Input: part model. Units: mm. Frame: model coordinates. Face numbers are marked on the shaded views. A direction names the side the tool comes from. Coordinates: 2 decimals unless noted, no trailing zeros. Order: outer loops, then holes, each group sorted by start corner. A loop starts at its lowest first (then second) coordinate and runs counter-clockwise, first axis right, second up. Notation, with made-up numbers: (3.5, -28.75) -> (30.5, -28.75) arc R18 ccw to (30.5, -16.75) -> close; hole circle Ø7 at (20.5, 5). An arc over 180 degrees is marked (long way). One line per item, written item: value. Start each with the question number.
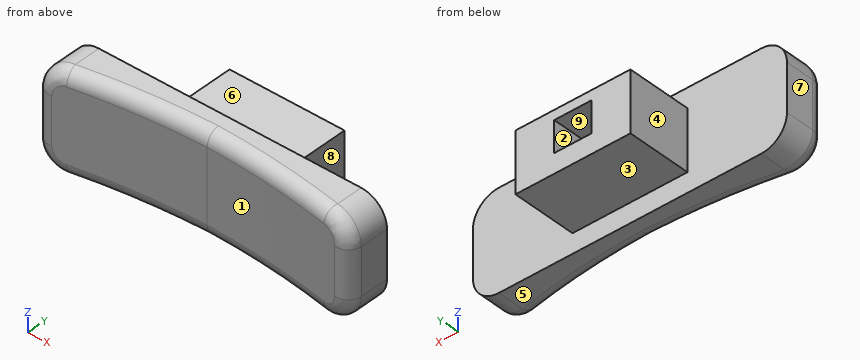
Autodesk Inventor part; units mm, degrees
ref_plane "Work Plane1" through (65.3719, 0, -59.3656) normal (0, 0, -1) x (-1, 0, 0)
ref_plane "Work Plane2" through (64.6469, 0, -58.7656) normal (1, 0, 0) x (0, 0, -1)
ref_plane "YZ Plane" through (0, 0, 0) normal (1, 0, 0) x (0, 1, 0)
sketch "Sketch3" plane through (0, 0, 0) normal (0, 1, 0) x (-1, 0, 0)
  line L0 (-64.0219, -58.8656) -> (-65.2719, -58.8656)
  line L1 (-65.2719, -58.8656) -> (-65.2719, -59.8656)
  line L2 (-65.2719, -59.8656) -> (-64.0219, -59.8656)
  line L3 (-64.0219, -59.8656) -> (-64.0219, -58.8656)
  line L4 (-63.9219, -59.9656) -> (-65.3719, -59.9656)
  line L5 (-65.3719, -59.9656) -> (-65.3719, -58.7656)
  line L6 (-65.3719, -58.7656) -> (-63.9219, -58.7656)
  line L7 (-63.9219, -58.7656) -> (-63.9219, -59.9656)
  line L8 (-66.8719, -60.7156) -> (-62.4219, -60.7156)
  line L9 (-62.4219, -60.7156) -> (-62.4219, -58.3956)
  line L10 (-62.4219, -58.3956) -> (-66.8719, -58.3956)
  line L11 (-66.8719, -58.3956) -> (-66.8719, -60.7156)
  line L12 (-70.1719, -61.0956) -> (-70.1719, -58.0956)
  line L13 (-70.1719, -58.0956) -> (-60.6119, -58.0956)
  line L14 (-60.6119, -61.0956) -> (-60.6119, -58.0956)
  dimension "d4" = 0.1
  dimension "d8" = 1.5
  dimension "d9" = 1.5
  dimension "d10" = 0.3
  dimension "d11" = 0.75
extrude "Extrusion3" add sketch "Sketch3" along normal blind 2.5 contours L11 L10 L9 L8
ref_plane "Work Plane1" through (65.3719, 0, -59.3656) normal (0, 0, -1) x (-1, 0, 0)
ref_plane "Work Plane2" through (64.6469, 0, -58.7656) normal (1, 0, 0) x (0, 0, -1)
sketch "Sketch4" plane through (0, 0, 0) normal (0, -1, 0) x (1, 0, 0)
  line L0 (60.1219, -61.0956) -> (60.1219, -58.0956)
  line L1 (67.6819, -58.0956) -> (67.6819, -61.0956)
  line L2 (60.1219, -58.0956) -> (67.6819, -58.0956)
  line L3 (62.4219, -58.3956) -> (66.8719, -58.3956)
  line L4 (66.8719, -58.3956) -> (66.8719, -60.7156)
  line L5 (66.8719, -60.7156) -> (62.4219, -60.7156)
  line L6 (62.4219, -60.7156) -> (62.4219, -58.3956)
  line L7 (70.7219, -57.6456) -> (58.5719, -57.6456)
  line L8 (58.5719, -57.6456) -> (58.5719, -61.4656)
  line L9 (58.5719, -61.4656) -> (70.7219, -61.4656)
  line L10 (70.7219, -61.4656) -> (70.7219, -57.6456)
  dimension "d13" = 3.85
  dimension "d14" = 3.85
extrude "Extrusion4" add sketch "Sketch4" along normal blind 1 contours L3 L4 L5 L6 | L10 L9 L8 L7
fillet "Fillet1" radius 1 4 edges at (70.7219, -0.5, -61.4656) (58.5719, -0.5, -61.4656) (58.5719, -0.5, -57.6456) (70.7219, -0.5, -57.6456)
sketch "Sketch6" plane through (69.7219, 0, -61.4656) normal (0, 0, -1) x (-1, 0, 0)
  line L0 (10.15, -1) -> (0, -1)
  line L1 (11.15, -1) -> (10.15, -1)
  line L2 (0, -1) -> (-1, -1)
  line L3 (11.15, -1) -> (11.15, -1.75)
  line L4 (0, -1) -> (10.15, -1)
  line L5 (5.075, -1) -> (5.075, -2.2009)
  arc A0 (11.15, -1.75) -> (5.075, -1) centre (4.574, -30.0368) ccw
  line L6 (-1, -1) -> (-1, -1.75)
  arc A1 (5.075, -1) -> (-1, -1.75) centre (5.576, -30.0368) ccw
  dimension "d18" = 0.75
extrude "Extrusion5" add sketch "Sketch6" against normal up to surface (3.82 mm away)
sketch "Sketch7" plane through (69.7219, -1, -61.4656) normal (0, 1, 0) x (1, 0, 0)
  arc A0 (0, -3.82) -> (1, -2.82) centre (0, -2.82) ccw
  line L0 (0, -3.82) -> (1, -3.82)
  line L1 (1, -2.82) -> (1, -3.82)
  arc A1 (1, -1) -> (0, 0) centre (0, -1) ccw
  line L2 (1, 0) -> (1, -1)
  line L3 (0, 0) -> (1, 0)
  arc A2 (-10.15, 0) -> (-11.15, -1) centre (-10.15, -1) ccw
  line L4 (-11.15, 0) -> (-10.15, 0)
  line L5 (-11.15, 0) -> (-11.15, -1)
  arc A3 (-11.15, -2.82) -> (-10.15, -3.82) centre (-10.15, -2.82) ccw
  line L6 (-11.15, -2.82) -> (-11.15, -3.82)
  line L7 (-11.15, -3.82) -> (-10.15, -3.82)
extrude "Extrusion6" cut sketch "Sketch7" against normal blind 1
fillet "Fillet2" radius 0.5 6 edges at (58.5719, -1.75, -59.5556) (62.0976, -1.1563, -57.6456) (62.0976, -1.1563, -61.4656) (70.7219, -1.75, -59.5556) (67.1962, -1.1563, -57.6456) (67.1962, -1.1563, -61.4656)
properties part number "Power Switch Cap"
1) Mould query, pull axis X, two halves, no side actions, for the marked faces 6, 7, 8 and 9. Classes: +X half, -X half, draft (parallel to the pull), parting line (faces both ways), or undercut.
2) Access query for the marked faces 1, 2, 3, 4 and 5. Directions: +Z, -Z, +X, -X, +Y, -Y. A direction counts if a zero-diameter tool reaches every point of the face in a straight line with its end or side. Return the directions, or none.
3) Pin query (flat end, axial travel): pin 1 Ø0.6 at (y, z) = (1, -59.5) entering from +X; pin 2 Ø1.2 at (y, z) = (1, -59) entering from -X. Return the tip coordinate at first contact, or that it passes through.
4) Section query A-A, the plane y = 0.3. Return the cut outline in (x, z).
5) Section query B-B, the plane z = -59.6. Return the cut outline in (x, y), plus the area to 3 significant figures.
6) Ray query, line 1 along Y through (x, z) = (70.25, -59.15); line 2 along X through (y, z) = (2, -59); line 3 along X through (y, z) = (0.1, -58.7). Return the intervals inside material, ascending. Write a range as from..to.
Entries:
1. face 6: draft
1. face 7: -X half
1. face 8: +X half
1. face 9: undercut
2. face 1: +Z, -Z, -Y
2. face 2: +Y
2. face 3: -Z, +X, -X, +Y
2. face 4: +Z, -Z, -X, +Y
2. face 5: -Z, +X, -X, +Y, -Y
3. pin 1: stops at x = 66.87
3. pin 2: stops at x = 62.42
4. outline: (62.42, -60.72) -> (66.87, -60.72) -> (66.87, -58.4) -> (62.42, -58.4) -> close; hole (63.92, -59.97) -> (65.37, -59.97) -> (65.37, -58.77) -> (63.92, -58.77) -> close
5. outline: (58.57, -1.13) arc R0.5 ccw to (59.17, -1.62) arc R29.04 cw to (64.65, -1) arc R29.04 cw to (70.12, -1.62) arc R0.5 ccw to (70.72, -1.13) -> (70.72, 0) -> (66.87, 0) -> (66.87, 2.5) -> (65.37, 2.5) -> (65.37, 0) -> (63.92, 0) -> (63.92, 2.5) -> (62.42, 2.5) -> (62.42, 0) -> (58.57, 0) -> close
5. area: 22.7 mm2
6. line 1: y = -1.63..0
6. line 2: x = 62.42..63.92, 65.37..66.87
6. line 3: x = 62.42..66.87
